from build123d import *

# Parameters (mm, degrees)
BOX001_W            = 5
BOX001_H            = 5
BOX001_DEPTH        = 5
CYLINDER157_R       = 2.25
CYLINDER157_DEPTH   = 7
CYLINDER156_R       = 1.2
CYLINDER156_DEPTH   = 14
CYLINDER147_R       = 1
CYLINDER147_DEPTH   = 1
ARRAY_COUNT         = 3
CYLINDER153_R       = 10
CYLINDER153_DEPTH   = 9
CUT_PLACEMENT_ANGLE = 180
CYLINDER158_R       = 3
CYLINDER158_DEPTH   = 23
CYLINDER_R          = 1
CYLINDER_DEPTH      = 10
CYLINDER159_R       = 4
CYLINDER159_DEPTH   = 20
BOX_W               = 22
BOX_H               = 22
BOX_DEPTH           = 9


with BuildPart() as cube001:
    # Box001 → Box001 (new body)
    with BuildSketch(Plane(origin=(5, -9, 3), x_dir=(1, 0, 0), z_dir=(0, 0, 1))):
        with Locations((2.5, 2.5)):
            Rectangle(BOX001_W, BOX001_H)
    extrude(amount=BOX001_DEPTH)


with BuildPart() as sealsubtraction:
    # Cylinder157 → Cylinder157 (new body)
    with BuildSketch(Plane.XY.offset(4.5)):
        Circle(CYLINDER157_R)
    extrude(amount=CYLINDER157_DEPTH)


with BuildPart() as bottomwireoutlet:
    # Cylinder156 → Cylinder156 (new body)
    with BuildSketch(Plane.XY.offset(-7)):
        Circle(CYLINDER156_R)
    extrude(amount=CYLINDER156_DEPTH)


with BuildPart() as sealarray:
    # Cylinder147 → Cylinder147 (new body)
    with BuildSketch(Plane.XY.offset(4.5)):
        Circle(CYLINDER147_R)
    extrude(amount=CYLINDER147_DEPTH)

    # Fusion: union SealSubtraction, BottomWireOutlet
    add(sealsubtraction.part)
    add(bottomwireoutlet.part)


with BuildPart() as sealarray_1:
    # Fusion placement: moved
    add(sealarray.part.moved(Location((4.25, 0, 0))))

    # Array: SealArray ×3 about axis
    array_axis = Axis((0, 0, 0), (0, 0, 1))


with BuildPart() as sealarray_2:
    add(sealarray_1.part)
    for i in range(1, ARRAY_COUNT):
        add(sealarray_1.part.rotate(array_axis, i * 360 / ARRAY_COUNT))


with BuildPart() as cut:
    # Cylinder153 → Cylinder153 (new body)
    with BuildSketch(Plane.XY.offset(-1)):
        Circle(CYLINDER153_R)
    extrude(amount=CYLINDER153_DEPTH)

    # Cut: cut SealArray
    add(sealarray_2.part, mode=Mode.SUBTRACT)


with BuildPart() as cut_1:
    # Cut placement: moved
    add(cut.part.moved(Location((0, 0, 9))).rotate(Axis((0, 0, 9), (1, 0, 0)), CUT_PLACEMENT_ANGLE))


with BuildPart() as cylinder001:
    # Cylinder158 → Cylinder158 (new body)
    with BuildSketch(Plane(origin=(10, -10, 3), x_dir=(1, 0, 0), z_dir=(0, 0, 1))):
        Circle(CYLINDER158_R)
    extrude(amount=CYLINDER158_DEPTH)


with BuildPart() as fusion003:
    # Cylinder → Cylinder (new body)
    with BuildSketch(Plane.XY.offset(6)):
        Circle(CYLINDER_R)
    extrude(amount=CYLINDER_DEPTH)

    # Fusion001: union Cylinder001
    add(cylinder001.part)

    # Fusion003: union Cut
    add(cut_1.part)


with BuildPart() as cylinder002:
    # Cylinder159 → Cylinder159 (new body)
    with BuildSketch(Plane(origin=(10, -10, 0), x_dir=(1, 0, 0), z_dir=(0, 0, 1))):
        Circle(CYLINDER159_R)
    extrude(amount=CYLINDER159_DEPTH)


with BuildPart() as cut002:
    # Box → Box (new body)
    with BuildSketch(Plane(origin=(-11, -11, 0), x_dir=(1, 0, 0), z_dir=(0, 0, 1))):
        with Locations((11, 11)):
            Rectangle(BOX_W, BOX_H)
    extrude(amount=BOX_DEPTH)

    # Fusion002: union Cylinder002
    add(cylinder002.part)

    # Cut001: cut Fusion003
    add(fusion003.part, mode=Mode.SUBTRACT)

    # Cut002: cut Cube001
    add(cube001.part, mode=Mode.SUBTRACT)


solid = cut002.part
Model file for the job. Use its own axes, mm. A direction names the side the tool comes from. Round coordinates to 2 decimals unless told otherwise and drop trailing zeros. Loops run counter-clockwise (first coordinate to the right, second up) from the corner with the lowest first, then second, coordinate; pieces in that order, holes last. Notation, with made-up numbers: M 19.5,35 L 23.5,35 A23 ccw 23.5,60 Z; hole C 33,54 d6. An arc over 180 degrees is marked long. One line per question, with ' | ' between items.
1) Band-saw the part on A-A (y = 0). Give the cut face in (x, z), then the cut area to 4 significant figures.
Solved:
outline: M -11,0 L 11,0 L 11,9 L 10,9 L 10,1 L 6.5,1 L 6.5,4.5 L 5.45,4.5 L 5.45,9 L 3.05,9 L 3.05,4.5 L 2,4.5 L 2,1 L -10,1 L -10,9 L -11,9 Z | area: 64.55 mm²
2) Drill centre lines: line 1 along Y through (x, z) = (0, 5.75); line 2 along X through (y, z) = (4.5, 8.25); line 3 along X through (y, z) = (-3.25, 3). Where is each one in solid material? Low to high.
Solved:
line 1: y = -11 to -10, 10 to 11 | line 2: x = -11 to -8.93, -3 to -1.25, 8.93 to 11 | line 3: x = -11 to -9.46, -4.33 to 0.08, 9.46 to 11
3) Band-saw the part on D-D (x = 4.25). Give the cut face in (y, z), then the cut area to 3 significant figures.
Solved:
outline: M -11,0 L 11,0 L 11,9 L 9.05,9 L 9.05,1 L 2.25,1 L 2.25,4.5 L 1.2,4.5 L 1.2,9 L -1.2,9 L -1.2,4.5 L -2.25,4.5 L -2.25,1 L -9.05,1 L -9.05,9 L -11,9 Z | area: 79.7 mm²
4) 3-axis set-ups, long thin cutter, end or side, ignore diameter. For faces 1 (the cylindrical face through (-2.39, 4.85, 6.78)), 2 (the flat face through (-2, -4, 9)), 3 (the flat face through (8, -7, 8)), 4 (the flat face through (-3, -11, 4)): which of +Z, -Z, +X, -X, +Y, -Y reach the whole face in a straight line?
Solved:
face 1: +Z | face 2: +Z, +X, -X, +Y, -Y | face 3: none | face 4: +Z, -Z, -X, -Y
5) Flat gauge pins, fed straight in: pin 1 (0.7 mm diameter, centred on x = 4, y = -0.5, fed in from +Z); pin 2 (3 mm diameter, centred on x = -7, z = 7, fed in from -Y); pin 3 (4 mm diameter, centred on y = -3, z = 7, fed in from +X). Where does each tip first touch, or does it go through?
Solved:
pin 1: stops at z = 9 | pin 2: stops at y = -11 | pin 3: stops at x = 11
6) Mould opens along X. For faces 5 (the flat face through (10, -9, 3)), 6 (the flat face through (-11, 0, 4)), 7 (the flat face through (4, 0, 9)), 8 (the flat face through (11, 2, 4)) say: +X half, -X half, draft (parallel to the pull), parting line (faces both ways), or undercut.
Solved:
face 5: undercut | face 6: -X half | face 7: draft | face 8: +X half
7) Band-saw the part on B-B (z = 3.75). Give the cut face in (x, y) (3 decimals), then the cut area to 3 significant figures.
Solved:
outline: M -11,-11 L 6.127,-11 A4 ccw long 11,-6.127 L 11,11 L -11,11 Z; C -2.125,-3.681 d4.5; C -2.125,3.681 d4.5; C 4.25,0 d4.5; hole M 5,-9 L 7.172,-9 A3 ccw long 10,-7 L 10,-4 L 9.165,-4 A10 ccw long 5,-8.66 Z | area: 209 mm²
8) Band-saw the part on C-C (x = 8.5). Give the cut face in (y, z).
Solved:
outline: M -13.71,0 L 11,0 L 11,9 L 5.27,9 L 5.27,1 L -5.27,1 L -5.27,3 L -12.6,3 L -12.6,20 L -13.71,20 Z; M -7.4,8 L -5.27,8 L -5.27,9 L -6.29,9 L -6.29,20 L -7.4,20 Z
